Verification items for the finished model (mm, model axes). Face numbers are marked on the shaded views. A direction names the side the tool comes from. Give positions to 0.01 mm unless a question says otherwise; leave off trailing zeros. Order: outer loops, then holes, each group sorted by start corner. A loop starts at its lowest first (then second) coordinate and runs counter-clockwise, first axis right, second up.
Autodesk Fusion 360 part; units mm, degrees
sketch "Face" plane through (0, 0, 0) normal (0, 0, 1) x (1, 0, 0)
  line L0 (0, 0) -> (120.02, 0) construction
  line L1 (120.02, 0) -> (120.02, 21.59) construction
  line L2 (120.02, 21.59) -> (0, 21.59) construction
  line L3 (0, 21.59) -> (0, 6.655) construction
  line L4 (120.02, 2.54) -> (116.52, 2.54)
  line L5 (120.02, 21.59) -> (116.52, 21.59)
  line L6 (116.52, 2.54) -> (113.98, 0)
  line L7 (116.52, 2.54) -> (120.1121, 2.54) construction
  line L8 (116.52, 21.59) -> (113.35, 18.42)
  line L9 (116.52, 21.59) -> (120.02, 21.59) construction
  line L10 (113.35, 18.42) -> (11.1657, 18.42)
  line L11 (11.1657, 0) -> (7.0507, 4.115)
  line L12 (11.1657, 0) -> (18.2593, 0) construction
  line L13 (11.1657, 18.42) -> (7.0507, 14.305)
  line L14 (11.1657, 18.42) -> (18.3401, 18.42) construction
  line L15 (7.24, 21.59) -> (7.24, 0) construction
  line L16 (0, 9.21) -> (7.24, 9.21) construction
  line L17 (0, 9.21) -> (0, 14.305) construction
  line L18 (0, 9.21) -> (0, 4.115) construction
  line L19 (2.54, 14.305) -> (7.0507, 14.305)
  line L20 (2.54, 4.115) -> (7.0507, 4.115)
  line L21 (0, 9.21) -> (13.01, 9.21) construction
  line L22 (11.1657, 0) -> (113.98, 0)
  line L23 (120.02, 21.59) -> (120.02, 2.54)
  arc A0 (2.54, 14.305) -> (0, 11.765) centre (2.54, 11.765) ccw
  arc A1 (0, 6.655) -> (2.54, 4.115) centre (2.54, 6.655) ccw
  line L24 (0, 11.765) -> (0, 6.655)
  line L25 (0, 9.21) -> (30.5, 9.21) construction
  line L26 (0, 9.21) -> (54.3, 9.21) construction
  line L27 (30.5, 0) -> (30.5, 21.59) construction
  line L28 (45.75, 0) -> (45.75, 21.59) construction
  line L29 (54.3, 9.21) -> (69.55, 9.21) construction
  line L30 (27.75, 18.42) -> (27.75, 0) construction
  line L31 (27.75, 14.62) -> (30.5, 14.62) construction
  circle A2 centre (27.75, 14.62) radius 1.625
  line L32 (27.75, 9.57) -> (30.5, 9.57) construction
  circle A3 centre (27.75, 9.57) radius 1.625
  line L33 (69.55, 9.21) -> (69.55, 18.42) construction
  line L34 (30.5, 18.42) -> (69.55, 18.42) construction
  line L35 (69.55, 18.42) -> (69.55, 15.72) construction
  line L36 (69.55, 15.72) -> (30.5, 15.72) construction
  line L37 (30.5, 15.72) -> (30.5, 18.42) construction
  line L38 (30.5, 15.72) -> (45.75, 15.72)
  line L39 (45.75, 15.72) -> (45.75, 4.72)
  line L40 (45.75, 4.72) -> (30.5, 4.72)
  line L41 (30.5, 4.72) -> (30.5, 15.72)
  line L42 (69.55, 15.72) -> (54.3, 15.72)
  line L43 (54.3, 15.72) -> (54.3, 4.72)
  line L44 (54.3, 4.72) -> (69.55, 4.72)
  line L45 (69.55, 4.72) -> (69.55, 15.72)
  circle A4 centre (51.55, 14.62) radius 1.625
  circle A5 centre (51.55, 9.57) radius 1.625
  dimension "d1" = 120.02
  dimension "d2" = 21.59
  dimension "d3" = 19.05
  dimension "d4" = 3.5
  dimension "d6" = 135
  dimension "d7" = 135
  dimension "d8" = 18.42
  dimension "d9" = 135
  dimension "d10" = 135
  dimension "d13" = 9.21
  dimension "d14" = 5.095
  dimension "d15" = 5.095
  dimension "d16" = 10.19
  dimension "d17" = 13.01
  dimension "d35" = 2.54
  dimension "d36" = 2.54
  dimension "d37" = 30.5
  dimension "d38" = 54.3
  dimension "d39" = 15.25
  dimension "d42" = 15.25
  dimension "d45" = 2.75
  dimension "d46" = 3.8
  dimension "d47" = 3.25
  dimension "d48" = 8.85
  dimension "d49" = 3.25
  dimension "d51" = 2.7
  dimension "d52" = 11
  dimension "d53" = 11
  dimension "d54" = 3.25
  dimension "d55" = 3.25
ref_plane "WorkPlane1" through (120.02, 0, 0) normal (1, 0, 0) x (0, 1, 0)
sketch "Arm" plane through (120.02, 0, 0) normal (1, 0, 0) x (0, 1, 0)
  line L0 (0, 0) -> (21.59, 0) construction
  line L1 (21.59, 0) -> (21.59, 12.23) construction
  line L2 (19.05, 12.23) -> (5.08, 12.23) construction
  line L3 (0, 12.23) -> (0, 0) construction
  line L4 (0, 0) -> (2.54, 0) construction
  line L5 (2.54, 0) -> (2.54, 11.43) construction
  line L6 (2.54, 11.43) -> (0, 11.43) construction
  line L7 (0, 11.43) -> (0, 0) construction
  line L8 (21.59, 12.23) -> (18.41, 12.23) construction
  line L9 (18.41, 12.23) -> (18.41, 0) construction
  line L10 (18.41, 5.88) -> (21.59, 5.88) construction
  line L11 (21.59, 5.88) -> (21.59, 12.23) construction
  line L12 (2.54, 9.69) -> (2.54, 0)
  line L13 (2.54, 0) -> (21.59, 0)
  line L14 (18.41, 8.09) -> (21.5902, 8.09)
  line L15 (18.41, 3.67) -> (21.594, 3.67)
  arc A0 (18.41, 8.09) -> (18.41, 3.67) centre (18.41, 5.88) ccw
  line L16 (2.54, 12.23) -> (10.92, 12.23) construction
  line L17 (10.92, 12.23) -> (10.92, 0) construction
  line L18 (10.92, 0) -> (2.54, 0) construction
  line L19 (2.54, 0) -> (2.54, 12.23) construction
  line L20 (10.92, 12.23) -> (13.97, 12.23) construction
  line L21 (13.97, 12.23) -> (13.97, 0) construction
  line L22 (13.97, 0) -> (10.92, 0) construction
  line L23 (10.92, 0) -> (10.92, 12.23) construction
  line L24 (21.5902, 8.09) -> (2.54, 8.09) construction
  line L25 (10.92, 8.09) -> (13.97, 8.09)
  line L26 (13.97, 8.09) -> (13.97, 12.23)
  line L27 (21.59, 12.23) -> (13.97, 12.23)
  line L28 (10.92, 12.23) -> (2.54, 12.23)
  line L29 (13.97, 8.09) -> (16.3602, 12.23)
  line L30 (13.97, 8.09) -> (18.4336, 8.09) construction
  line L31 (10.92, 8.09) -> (8.5298, 12.23)
  line L32 (10.92, 8.09) -> (15.5777, 8.09) construction
  line L33 (21.59, 0) -> (21.59, 3.67)
  line L34 (21.59, 8.09) -> (21.59, 9.69)
  arc A1 (21.59, 9.69) -> (19.05, 12.23) centre (19.05, 9.69) ccw
  arc A2 (5.08, 12.23) -> (2.54, 9.69) centre (5.08, 9.69) ccw
  line L35 (0, 0) -> (2.54, 0)
  line L36 (2.54, 0) -> (2.54, 0.8)
  line L37 (2.54, 0.8) -> (0, 0.8)
  line L38 (0, 0.8) -> (0, 0)
  line L39 (10.92, 8.09) -> (10.92, 12.23)
  line L40 (2.54, 0.8) -> (21.59, 0.8016) construction
  dimension "d20" = 21.59
  dimension "d21" = 12.23
  dimension "d22" = 2.54
  dimension "d23" = 3.18
  dimension "d24" = 6.35
  dimension "d25" = 4.42
  dimension "d26" = 8.38
  dimension "d27" = 3.05
  dimension "d28" = 60
  dimension "d29" = 120
  dimension "d30" = 2.54
  dimension "d31" = 2.54
  dimension "d32" = 2.54
  dimension "d33" = 0.8
  dimension "d34" = 11.43
ref_plane "WorkPlane2" through (0, 18.42, 0) normal (0, 1, 0) x (0, 0, 1)
sketch "Tabs" plane through (0, 18.42, 0) normal (0, 1, 0) x (1, 0, 0)
  line L0 (0, 0) -> (23.75, 0) construction
  line L1 (23.75, 0) -> (23.75, 13.05) construction
  line L2 (22.5, 14.3) -> (17.5, 14.3) construction
  line L3 (0, 14.3) -> (0, 0) construction
  line L4 (23.75, 0) -> (16.25, 0)
  line L5 (16.25, 0) -> (16.25, 13.05)
  line L6 (16.25, 14.3) -> (22.5, 14.3)
  line L7 (23.75, 13.05) -> (23.75, 0)
  line L8 (70.75, 0) -> (70.75, 13.05)
  line L9 (72, 14.3) -> (77, 14.3)
  line L10 (78.25, 13.05) -> (78.25, 0)
  line L11 (78.25, 0) -> (70.75, 0)
  line L12 (16.25, 11.325) -> (23.75, 11.325) construction
  line L13 (0, 0) -> (120.02, 0)
  circle A0 centre (20, 11.325) radius 1.325
  circle A1 centre (74.5, 11.325) radius 1.325
  arc A2 (17.5, 14.3) -> (16.25, 13.05) centre (17.5, 13.05) ccw
  arc A3 (72, 14.3) -> (70.75, 13.05) centre (72, 13.05) ccw
  arc A4 (78.25, 13.05) -> (77, 14.3) centre (77, 13.05) ccw
  arc A5 (23.75, 13.05) -> (22.5, 14.3) centre (22.5, 13.05) ccw
  line L14 (23.75, 13.05) -> (23.75, 14.3) construction
  line L15 (22.5, 14.3) -> (23.75, 14.3) construction
  dimension "d57" = 23.75
  dimension "d58" = 14.3
  dimension "d59" = 7.5
  dimension "d60" = 7.5
  dimension "d62" = 54.5
  dimension "d63" = 85.75
  dimension "d64" = 11.325
  dimension "d65" = 2.65
  dimension "d66" = 2.65
  dimension "d67" = 1.25
  dimension "d69" = 1.25
  dimension "d70" = 1.25
  dimension "d79" = 1.25
extrude "Extrude1" add sketch "Face" along normal blind 0.5
extrude "Extrude2" add sketch "Arm" along normal blind 0.8 contours L12 L13 L14 L15 A0 L25 L27 L28 L29 L31 L33 L34 A1 A2 L36 | L28 L31 L39 | L26 L27 L29
extrude "Extrude3" add sketch "Tabs" against normal blind 0.8 contours L8 L9 L10 L11 L13 A3 A4
extrude "Extrude4" add sketch "Tabs" against normal blind 0.8 contours L4 L5 L6 L7 L13 A2 A5
sketch "Sketch5" plane through (0, 0, 0) normal (0, 1, 0) x (1, 0, 0)
  line L0 (0, 0) -> (113.98, 0) construction
  line L1 (113.98, 0) -> (113.98, 2.54) construction
  line L2 (113.98, 2.54) -> (0, 2.54) construction
  line L3 (0, 2.54) -> (0, 0) construction
  line L4 (11.166, 0) -> (11.166, 2.54) construction
  line L5 (16.246, 0) -> (16.246, 2) construction
  line L6 (111.44, 0) -> (111.44, 1.54) construction
  line L7 (16.246, 0) -> (111.44, 0)
  line L8 (111.44, 0) -> (111.44, 2.54)
  line L9 (110.44, 2.54) -> (17.246, 2.54)
  line L10 (16.246, 1.54) -> (16.246, 0)
  arc A0 (17.246, 2.54) -> (16.246, 1.54) centre (17.246, 1.54) ccw
  arc A1 (111.44, 1.54) -> (110.44, 2.54) centre (110.44, 1.54) ccw
  dimension "d86" = 113.98
  dimension "d87" = 2.54
  dimension "d88" = 11.166
  dimension "d89" = 5.08
  dimension "d90" = 2.54
  dimension "d91" = 1
  dimension "d92" = 1
extrude "Extrude5" add sketch "Sketch5" along normal blind 0.8
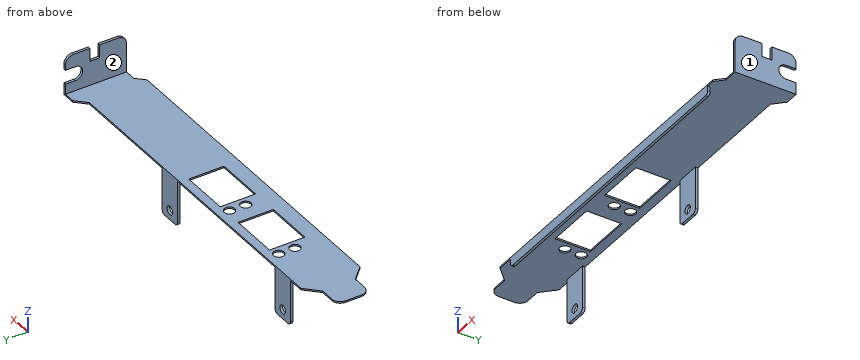
(1) Section check D-D, the plane y = 20.25. Enter the section's corners in (x, z).
Solved:
outline: (115.18, 0) - (120.82, 0) - (120.82, 3.67) - (120.02, 3.67) - (120.02, 0.5) - (115.18, 0.5) - close; (120.02, 8.09) - (120.82, 8.09) - (120.82, 11.93) - (120.02, 11.93) - close
(2) Go/stop test with flat-tipped pins: pin 1 (4 mm diameter, centred on x = 74, z = -8, fed in from -Y); pin 2 (0.6 mm diameter, centred on x = 61.5, z = 0, fed in from +Y); pin 3 (2 mm diameter, centred on x = 73, y = 18.5, fed in from +Z); pin 4 (8 mm diameter, centred on x = 106, z = -1.5, fed in from -Y). Record where each tip stops, or that it passes through.
Solved:
pin 1: stops at y = 17.62
pin 2: stops at y = 18.42
pin 3: stops at z = 0.5
pin 4: stops at y = 0
(3) Set-up check for the marked faces 1 and 2: record each of +Z, -Z, +X, -X, +Y, -Y from which the full face is reachable in a straight line by a thin tool's end or side.
Solved:
face 1: +Z, -Z, +X, +Y, -Y
face 2: +Z, -X, +Y, -Y
(4) Section check B-B, the plane z = -5.5. Enter the section's corners in (x, y).
Solved:
outline: (16.25, 17.62) - (23.75, 17.62) - (23.75, 18.42) - (16.25, 18.42) - close; (70.75, 17.62) - (78.25, 17.62) - (78.25, 18.42) - (70.75, 18.42) - close
(5) Section check C-C, the plane x = 27.75. Enter the section's corners in (y, z) (3 decimals).
Solved:
outline: (0, -2.54) - (0.8, -2.54) - (0.8, 0) - (7.945, 0) - (7.945, 0.5) - (0, 0.5) - close; (11.195, 0) - (12.995, 0) - (12.995, 0.5) - (11.195, 0.5) - close; (16.245, 0) - (18.42, 0) - (18.42, 0.5) - (16.245, 0.5) - close
(6) Section check A-A, the plane x = 74.5. Enter the section's corners in (y, z).
Solved:
outline: (0, -2.54) - (0.8, -2.54) - (0.8, 0) - (17.62, 0) - (17.62, -10) - (18.42, -10) - (18.42, 0.5) - (0, 0.5) - close; (17.62, -14.3) - (18.42, -14.3) - (18.42, -12.65) - (17.62, -12.65) - close
(7) Scan lines: line 1 (Z direction, x = 20, y = 18.25); line 2 (X direction, y = 3.5, z = 8.75); line 3 (Z direction, x = 58.5, y = 17.5). Record each from-to range of solid material in increasing order.
Solved:
line 1: z = -14.3 to -12.65, -10 to 0.5
line 2: x = 120.02 to 120.82
line 3: z = 0 to 0.5
